```python
from build123d import *

# Parameters (mm, degrees)
SKETCH1_W               = 74
SKETCH1_H               = 40
BOSS_EXTRUDE1_DEPTH     = 10
BOSS_EXTRUDE2_DEPTH     = 74
SKETCH3_R               = 1.75
CUT_EXTRUDE1_DEPTH      = 6
CUT_EXTRUDE1_DEPTH_BACK = 11
CUT_EXTRUDE2_DEPTH      = 6
CUT_EXTRUDE2_DEPTH_BACK = 3
FILLET1_R               = 1


with BuildPart() as part:
    # Sketch1 → Boss-Extrude1 (new body)
    with BuildSketch(Plane.XY):
        Rectangle(SKETCH1_W, SKETCH1_H)
    extrude(amount=BOSS_EXTRUDE1_DEPTH)

    # Sketch2 → Boss-Extrude2 (add)
    with BuildSketch(Plane.ZY.offset(37)):
        Polygon((10, 13.5), (10, 5.5), (15, 5.5), (15, 8.5), align=None)
        Polygon((15, -5.5), (10, -5.5), (10, -13.5), (15, -8.5), align=None)
    extrude(amount=-BOSS_EXTRUDE2_DEPTH)

    # Sketch3 → Cut-Extrude1 (cut, two sides)
    with BuildSketch(Plane.XY.offset(10)) as cut_extrude1_sk:
        with Locations((32.125, 15.125)):
            Circle(SKETCH3_R)
        with Locations((32.125, -15.125)):
            Circle(SKETCH3_R)
        with Locations((-32.125, -15.125)):
            Circle(SKETCH3_R)
        with Locations((-32.125, 15.125)):
            Circle(SKETCH3_R)
    extrude(amount=CUT_EXTRUDE1_DEPTH, mode=Mode.SUBTRACT)
    extrude(cut_extrude1_sk.sketch, amount=-CUT_EXTRUDE1_DEPTH_BACK, mode=Mode.SUBTRACT)

    # Sketch4 → Cut-Extrude2 (cut, two sides)
    with BuildSketch(Plane.XY.offset(10)) as cut_extrude2_sk:
        with BuildLine():
            Line((35.009956427, 15.428108891), (33.829978213, 17.471891109))
            ThreePointArc((33.829978213, 17.471891109), (33.829978213, 18.078108891), (33.304978213, 17.775))
            Line((33.304978213, 17.775), (30.945021787, 17.775))
            ThreePointArc((30.945021787, 17.775), (30.420021787, 18.078108891), (30.420021787, 17.471891109))
            Line((30.420021787, 17.471891109), (29.240043573, 15.428108891))
            ThreePointArc((29.240043573, 15.428108891), (28.715043573, 15.125), (29.240043573, 14.821891109))
            Line((29.240043573, 14.821891109), (30.420021787, 12.778108891))
            ThreePointArc((30.420021787, 12.778108891), (30.420021787, 12.171891109), (30.945021787, 12.475))
            Line((30.945021787, 12.475), (33.304978213, 12.475))
            ThreePointArc((33.304978213, 12.475), (33.829978213, 12.171891109), (33.829978213, 12.778108891))
            Line((33.829978213, 12.778108891), (35.009956427, 14.821891109))
            ThreePointArc((35.009956427, 14.821891109), (35.534956427, 15.125), (35.009956427, 15.428108891))
        make_face()
        with BuildLine():
            Line((-29.240043573, 15.428108891), (-30.420021787, 17.471891109))
            ThreePointArc((-30.420021787, 17.471891109), (-30.420021787, 18.078108891), (-30.945021787, 17.775))
            Line((-30.945021787, 17.775), (-33.304978213, 17.775))
            ThreePointArc((-33.304978213, 17.775), (-33.829978213, 18.078108891), (-33.829978213, 17.471891109))
            Line((-33.829978213, 17.471891109), (-35.009956427, 15.428108891))
            ThreePointArc((-35.009956427, 15.428108891), (-35.534956427, 15.125), (-35.009956427, 14.821891109))
            Line((-35.009956427, 14.821891109), (-33.829978213, 12.778108891))
            ThreePointArc((-33.829978213, 12.778108891), (-33.829978213, 12.171891109), (-33.304978213, 12.475))
            Line((-33.304978213, 12.475), (-30.945021787, 12.475))
            ThreePointArc((-30.945021787, 12.475), (-30.420021787, 12.171891109), (-30.420021787, 12.778108891))
            Line((-30.420021787, 12.778108891), (-29.240043573, 14.821891109))
            ThreePointArc((-29.240043573, 14.821891109), (-28.715043573, 15.125), (-29.240043573, 15.428108891))
        make_face()
        with BuildLine():
            Line((-29.240043573, -14.821891109), (-30.420021787, -12.778108891))
            ThreePointArc((-30.420021787, -12.778108891), (-30.420021787, -12.171891109), (-30.945021787, -12.475))
            Line((-30.945021787, -12.475), (-33.304978213, -12.475))
            ThreePointArc((-33.304978213, -12.475), (-33.829978213, -12.171891109), (-33.829978213, -12.778108891))
            Line((-33.829978213, -12.778108891), (-35.009956427, -14.821891109))
            ThreePointArc((-35.009956427, -14.821891109), (-35.534956427, -15.125), (-35.009956427, -15.428108891))
            Line((-35.009956427, -15.428108891), (-33.829978213, -17.471891109))
            ThreePointArc((-33.829978213, -17.471891109), (-33.829978213, -18.078108891), (-33.304978213, -17.775))
            Line((-33.304978213, -17.775), (-30.945021787, -17.775))
            ThreePointArc((-30.945021787, -17.775), (-30.420021787, -18.078108891), (-30.420021787, -17.471891109))
            Line((-30.420021787, -17.471891109), (-29.240043573, -15.428108891))
            ThreePointArc((-29.240043573, -15.428108891), (-28.715043573, -15.125), (-29.240043573, -14.821891109))
        make_face()
        with BuildLine():
            Line((35.009956427, -14.821891109), (33.829978213, -12.778108891))
            ThreePointArc((33.829978213, -12.778108891), (33.829978213, -12.171891109), (33.304978213, -12.475))
            Line((33.304978213, -12.475), (30.945021787, -12.475))
            ThreePointArc((30.945021787, -12.475), (30.420021787, -12.171891109), (30.420021787, -12.778108891))
            Line((30.420021787, -12.778108891), (29.240043573, -14.821891109))
            ThreePointArc((29.240043573, -14.821891109), (28.715043573, -15.125), (29.240043573, -15.428108891))
            Line((29.240043573, -15.428108891), (30.420021787, -17.471891109))
            ThreePointArc((30.420021787, -17.471891109), (30.420021787, -18.078108891), (30.945021787, -17.775))
            Line((30.945021787, -17.775), (33.304978213, -17.775))
            ThreePointArc((33.304978213, -17.775), (33.829978213, -18.078108891), (33.829978213, -17.471891109))
            Line((33.829978213, -17.471891109), (35.009956427, -15.428108891))
            ThreePointArc((35.009956427, -15.428108891), (35.534956427, -15.125), (35.009956427, -14.821891109))
        make_face()
    extrude(amount=CUT_EXTRUDE2_DEPTH, mode=Mode.SUBTRACT)
    extrude(cut_extrude2_sk.sketch, amount=-CUT_EXTRUDE2_DEPTH_BACK, mode=Mode.SUBTRACT)

    # Fillet1
    fillet1_edges = [part.edges().sort_by_distance(p)[0] for p in [
        (-37, 16.75, 10),
        (37, 16.75, 10),
        (-37, 0, 10),
        (0, 8.5, 15),
        (0, 5.5, 15),
        (0, 5.5, 10),
        (0, -20, 10),
        (35.62338112, 13.5, 10),
        (-37, 7, 15),
        (-37, 11, 12.5),
        (-37, 5.5, 12.5),
        (37, 7, 15),
        (37, 5.5, 12.5),
        (37, 11, 12.5),
        (37, 0, 10),
        (-37, -16.75, 10),
        (35.62338112, -13.5, 10),
        (37, -11, 12.5),
        (0, -8.5, 15),
        (-37, -11, 12.5),
        (37, -7, 15),
        (0, -5.5, 15),
        (-37, -7, 15),
        (37, -5.5, 12.5),
        (0, -5.5, 10),
        (-37, -5.5, 12.5),
        (37, -16.75, 10),
        (-35.62338112, -13.5, 10),
        (0, -13.5, 10),
        (-35.62338112, 13.5, 10),
        (0, 13.5, 10),
        (37, -20, 5),
        (-37, -20, 5),
        (-37, 20, 5),
        (37, 20, 5),
        (0, 20, 10),
    ]]
    fillet(fillet1_edges, radius=FILLET1_R)


solid = part.part
```
The listing builds one solid part. Answer for the finished solid, in the listing's coordinates (mm). A direction names the side the tool comes from. Coordinates: 2 decimals unless noted, no trailing zeros. Order: outer loops, then holes, each group sorted by start corner. A loop starts at its lowest first (then second) coordinate and runs counter-clockwise, first axis right, second up. Notation, with made-up numbers: M -25,-37 L -12,-37 A37 cw -12,-1 Z; hole C 77.5,-13.75 d8. An arc over 180 degrees is marked long. Answer as a JSON object with one key per item and string values. Group by question number.
1. Determine the mould class of faces 1 (the flat face through (-34.428, -16.436, 8.521)), 2 (the flat face through (-1, -16, 10)) for opening direction X: released by +X, released by -X, zero draft, split by the parting line, or undercut.
2. Flat-ended cylindrical pins translate along their axes: P1, Ø2.5, axis at x = -12, z = 12, coming from the +Y side; P2, Ø5.5, axis at x = 32.125, y = 15.125, coming from the +Z side (3 decimals); P3, Ø4, axis at x = 24.5, y = -16, coming from the +Z side. Find the tip coordinate at first contact, or state that the pin passes through.
3. Section B-B on x = 0 is taken. Write down the section's boundary in (y, z), then the cut area to 3 significant figures.
4. Straight lines are drawn through the part: line 1 (Y direction, x = 32, z = 5.25); line 2 (Z direction, x = 28, y = -12.5); line 3 (X direction, y = -16, z = 6.25). For each, find the intervals that lie inside material, in ascending order.
5. Section A-A on y = 2 is taken. Write down the section's boundary in (x, z), then the cut area to 3 significant figures.
6. A tool of negligible diameter and unlimited length cuts with its end or side. For faces 3 (the flat face through (-1, -5.5, 13)), 4 (the flat face through (-1, 20, 4)), 5 (the flat face through (-0.5, -11, 12.5)), 6 (the flat face through (-29.822, -13.814, 8.473)), 7 (the flat face through (-1, 16, 10)), from which of +Z, -Z, +X, -X, +Y, -Y can it reach the whole face along a straight path? Write none if from no direction.
Values follow:
{
 "1": {"face 1": "undercut", "face 2": "zero draft"},
 "2": {"P1": "y = 12.75", "P2": "z = 11.125", "P3": "z = 10"},
 "3": {"outline": "M -20,0 L 20,0 L 20,9 A1 ccw 19,10 L 13.91,10 A1 cw 13.21,10.29 L 8.79,14.71 A1 ccw 8.09,15 L 6.5,15 A1 ccw 5.5,14 L 5.5,11 A1 cw 4.5,10 L -4.5,10 A1 cw -5.5,11 L -5.5,14 A1 ccw -6.5,15 L -8.09,15 A1 ccw -8.79,14.71 L -13.21,10.29 A1 cw -13.91,10 L -19,10 A1 ccw -20,9 Z", "area": "455 mm2"},
 "4": {"line 1": "-20 to -16.87, -13.38 to 13.38, 16.87 to 20", "line 2": "0 to 11", "line 3": "-37 to -33.64, -30.61 to 30.61, 33.64 to 37"},
 "5": {"outline": "M -37,0 L 37,0 L 37,9 A1 ccw 36,10 L -36,10 A1 ccw -37,9 Z", "area": "740 mm2"},
 "6": {"face 3": "+Z, +X, -X", "face 4": "+Z, -Z, +X, -X, +Y", "face 5": "+Z, +X, -X, -Y", "face 6": "+Z", "face 7": "+Z, +X, -X, +Y"}
}
